Input: part model. Units: mm. Frame: model coordinates. A direction names the side the tool comes from. Round coordinates to 2 decimals unless told otherwise and drop trailing zeros. Write each loop counter-clockwise with the first axis right and the second up, starting at its lowest first coordinate (ties: lowest second). Pieces come first, ordered by that corner, then holes. Notation, with made-up numbers: (26, 24.25) - (43, 24.25) arc R13 ccw to (43, 30.25) - close; hole circle Ø5 at (81.5, -28.5). An arc over 180 degrees is marked (long way). One line per item, written item: value. Start each with the question number.
```python
from build123d import *

# Parameters (mm, degrees)
SKETCH2_R           = 1.1
SKETCH2_R_2         = 4.5
SKETCH2_R_3         = 1.55
BOSS_EXTRUDE1_DEPTH = 3.048


with BuildPart() as part:
    # Sketch2 → Boss-Extrude1 (new body)
    with BuildSketch(Plane(origin=(0, 0, 0), x_dir=(1, 0, 0), z_dir=(0, 1, 0))):
        with BuildLine():
            Line((3, 8), (71.45, 8))
            ThreePointArc((71.45, 8), (87.628603154, 1.298603154), (94.33, -14.88))
            Line((94.33, -14.88), (94.33, -71.310147445))
            ThreePointArc((94.33, -71.310147445), (90.950189058, -78.782657675), (83.340051803, -81.84))
            Line((83.340051803, -81.84), (3, -81.84))
            ThreePointArc((3, -81.84), (-4.778174593, -78.618174593), (-8, -70.84))
            Line((-8, -70.84), (-8, -3))
            ThreePointArc((-8, -3), (-4.778174593, 4.778174593), (3, 8))
        make_face()
        with Locations(Location((4.19, -71.01, 0), (0, 0, 90))):
            Circle(SKETCH2_R, mode=Mode.SUBTRACT)
        with Locations(Location((25.03, -71.01, 0), (0, 0, 90))):
            Circle(SKETCH2_R, mode=Mode.SUBTRACT)
        with Locations(Location((4.19, -2.98, 0), (0, 0, 90))):
            Circle(SKETCH2_R, mode=Mode.SUBTRACT)
        with Locations(Location((51.82, -2.98, 0), (0, 0, 90))):
            Circle(SKETCH2_R, mode=Mode.SUBTRACT)
        with Locations(Location((51.82, -26.2, 0), (0, 0, 90))):
            Circle(SKETCH2_R, mode=Mode.SUBTRACT)
        with Locations(Location((71.83, -14.33, 0), (0, 0, 90))):
            Circle(SKETCH2_R_2, mode=Mode.SUBTRACT)
        with Locations(Location((-2.656854249, 2.656854249, 0), (0, 0, 90))):
            Circle(SKETCH2_R_3, mode=Mode.SUBTRACT)
        with Locations(Location((85.50728281, -0.82271719, 0), (0, 0, 90))):
            Circle(SKETCH2_R_3, mode=Mode.SUBTRACT)
        with Locations(Location((88.858862501, -76.631761762, 0), (0, 0, 90))):
            Circle(SKETCH2_R_3, mode=Mode.SUBTRACT)
        with Locations(Location((-2.656854249, -76.496854249, 0), (0, 0, 90))):
            Circle(SKETCH2_R_3, mode=Mode.SUBTRACT)
        with BuildLine():
            Line((28, -66.24), (28, -32.84))
            ThreePointArc((28, -32.84), (28.878679656, -30.718679656), (31, -29.84))
            Line((31, -29.84), (83.33, -29.84))
            ThreePointArc((83.33, -29.84), (85.451320344, -30.718679656), (86.33, -32.84))
            Line((86.33, -32.84), (86.33, -66.24))
            ThreePointArc((86.33, -66.24), (85.451320344, -68.361320344), (83.33, -69.24))
            Line((83.33, -69.24), (31, -69.24))
            ThreePointArc((31, -69.24), (28.878679656, -68.361320344), (28, -66.24))
        make_face(mode=Mode.SUBTRACT)
        with BuildLine():
            Line((6.5, -6.84), (6.5, -57.34))
            ThreePointArc((6.5, -57.34), (6.353553391, -57.693553391), (6, -57.84))
            Line((6, -57.84), (3.5, -57.84))
            ThreePointArc((3.5, -57.84), (3.146446609, -57.693553391), (3, -57.34))
            Line((3, -57.34), (3, -6.84))
            ThreePointArc((3, -6.84), (3.146446609, -6.486446609), (3.5, -6.34))
            Line((3.5, -6.34), (6, -6.34))
            ThreePointArc((6, -6.34), (6.353553391, -6.486446609), (6.5, -6.84))
        make_face(mode=Mode.SUBTRACT)
        with BuildLine():
            Line((24.5, -6.84), (24.5, -57.34))
            ThreePointArc((24.5, -57.34), (24.353553391, -57.693553391), (24, -57.84))
            Line((24, -57.84), (21.5, -57.84))
            ThreePointArc((21.5, -57.84), (21.146446609, -57.693553391), (21, -57.34))
            Line((21, -57.34), (21, -6.84))
            ThreePointArc((21, -6.84), (21.146446609, -6.486446609), (21.5, -6.34))
            Line((21.5, -6.34), (24, -6.34))
            ThreePointArc((24, -6.34), (24.353553391, -6.486446609), (24.5, -6.84))
        make_face(mode=Mode.SUBTRACT)
    extrude(amount=BOSS_EXTRUDE1_DEPTH)


solid = part.part
```
Q1. Cut plane B-B, the plane x = 57. Output: boundary loops of the cut face in (y, z), and give its area (3 significant figures).
Q2. Pull-direction query (X, two-part tool) for faces 3 (the cylindrical face through (-4.692, 1.503, 78.703)), 4 (the cylindrical face through (28.9, 1.5, 30.7)), 5 (the cylindrical face through (91.035, 1.503, 78.701)), 6 (the flat face through (44, 0, 26)); classes: pulls with the +X half, pulls with the -X half, needs draft (parallel to the pull), parting line crosses it, or undercut.
Q3. Contact query for a flat-ended pin moving along its axis: pin 1 Ø14.5 at (x, z) = (71.83, 14.33) entering from -Y. Output: stop coordinate, or through.
Q4. Cut plane D-D, the plane z = 8. Output: boundary loops of the cut face in (x, y), and give its area (3 significant figures).
Q5. Material intervals for probe 1 along X at (y, z) = (0.95, 51.5); probe 2 along X at (y, z) = (2.4, 26.2); probe 3 along Z at (x, y) = (4.19, 1.3), sorted ascending. Write a range as from..to.
Q6. Cut plane C-C, the plane y = 1.6. Count the separate pieces of the cut face and the enclosed holes in it, and give its area (3 significant figures).
Q7. Cut plane A-A, the plane z = 21. Output: boundary loops of the cut face in (x, y).
Q8. Access query for faces 1 (the flat face through (23, 2, 6.34)), 2 (the flat face through (37, 2, -8)). Directions: +Z, -Z, +X, -X, +Y, -Y. A direction counts if a zero-diameter tool reaches every point of the face in a straight line with its end or side. Return the directions, or none.
A:
1. outline: (0, -8) - (3.05, -8) - (3.05, 29.84) - (0, 29.84) - close; (0, 69.24) - (3.05, 69.24) - (3.05, 81.84) - (0, 81.84) - close
1. area: 154 mm²
2. face 3: pulls with the -X half
2. face 4: undercut
2. face 5: pulls with the +X half
2. face 6: needs draft
3. pin 1: stops at y = 0
4. outline: (-8, 0) - (3, 0) - (3, 3.05) - (-8, 3.05) - close; (6.5, 0) - (21, 0) - (21, 3.05) - (6.5, 3.05) - close; (24.5, 0) - (93.27, 0) - (93.27, 3.05) - (24.5, 3.05) - close
4. area: 287 mm²
5. probe 1: x = -8..3, 6.5..21, 24.5..28, 86.33..94.33
5. probe 2: x = -8..3, 6.5..21, 24.5..50.72, 52.92..94.33
5. probe 3: z = -8..1.88, 4.08..6.34, 57.84..69.91, 72.11..81.84
6. separate pieces: 1
6. enclosed holes: 13
6. area: 6,240 mm²
7. outline: (-8, 0) - (3, 0) - (3, 3.05) - (-8, 3.05) - close; (6.5, 0) - (21, 0) - (21, 3.05) - (6.5, 3.05) - close; (24.5, 0) - (94.33, 0) - (94.33, 3.05) - (24.5, 3.05) - close
8. face 1: +Y, -Y
8. face 2: -Z, +X, -X, +Y, -Y
